Can you work these out from the model? Positions are in its coordinate system, mm. A direction names the side the tool comes from. Give positions to 0.01 mm unless a question says otherwise; leave off trailing zeros. Loops run counter-clockwise (first coordinate to the right, second up) from the corner with the lowest first, then second, coordinate; pieces in that order, holes last.
from build123d import *

# Parameters (mm, degrees)
F0_W     = 173
F0_H     = 30
F1_DEPTH = 3
F2_R     = 9
F3_DEPTH = 15
F4_R     = 2.5
F5_DEPTH = 25
F6_SIZE  = 1
F7_R     = 10
F7_R_2   = 9
F8_DEPTH = 1


with BuildPart() as f1:
    # F0 (on Top) → F1 (new body)
    with BuildSketch(Plane.XY):
        Rectangle(F0_W, F0_H)
    extrude(amount=-F1_DEPTH)

    # F2 (on face) → F3 (join)
    with BuildSketch(Plane.XY):
        with Locations((-67.5, 0.1318904841)):
            Circle(F2_R)
        with Locations((-22.5, 0.1318904841)):
            Circle(F2_R)
        with Locations((22.5, 0.1318904841)):
            Circle(F2_R)
        with Locations((67.5, 0.1318904841)):
            Circle(F2_R)
    extrude(amount=F3_DEPTH)

    # F4 (on face) → F5 (cut)
    with BuildSketch(Plane.XY):
        with Locations((-48.203933984, 0)):
            Circle(F4_R)
        with Locations((48.203933984, 0)):
            Circle(F4_R)
    extrude(amount=-F5_DEPTH, mode=Mode.SUBTRACT)

    # F6
    f6_edges = [f1.edges().sort_by_distance(p)[0] for p in [
        (-50.703934, 0, 0),
        (45.703934, 0, 0),
    ]]
    chamfer(f6_edges, length=F6_SIZE)

    # F7 (on face) → F8 (join, symmetric)
    with BuildSketch(Plane.XY.offset(15)):
        with Locations((-67.5, 0.1318904841)):
            Circle(F7_R)
        with Locations((-67.5, 0.1318904841)):
            Circle(F7_R_2, mode=Mode.SUBTRACT)
        with Locations((-22.5, 0.1318904841)):
            Circle(F7_R)
        with Locations((22.5, 0.1318904841)):
            Circle(F7_R)
        with Locations((67.5, 0.1318904841)):
            Circle(F7_R)
        with Locations((-67.5, 0.1318904841)):
            Circle(F7_R_2)
    extrude(amount=F8_DEPTH, both=True)


solid = f1.part
(1) Which directions (+Z, -Z, +X, -X, +Y, -Y) give clear straight access to the entire face, cutting with the end or side of a thin tool? Please do faces 4 (the flat face through (86.5, 0, -1)), 5 (the cylindrical face through (76.084, 2.835, 6.902)), 6 (the cylindrical face through (-77.49, 0.57, 15.01)).
Returned:
face 4: +Z, -Z, +X, +Y, -Y
face 5: none
face 6: +Z
(2) Will these pins go through, and if not, where does the flat tip stop? P1, Ø6, axis at y = 8.5, z = 10.5, coming from the +X side; P2, Ø15, axis at x = -0.5, y = 5.5, coming from the +Z side; P3, Ø4, axis at x = 25, z = 9, coming from the -Y side.
Returned:
P1: stops at x = 74.72
P2: stops at z = 0
P3: stops at y = -8.85
(3) Suppose I cut it at D-D on x = -29. List the corners of the cut face in (y, z) for me, plus the area to 3 significant figures.
Returned:
outline: (-15, -3) - (15, -3) - (15, 0) - (6.36, 0) - (6.36, 14) - (7.73, 14) - (7.73, 16) - (-7.47, 16) - (-7.47, 14) - (-6.09, 14) - (-6.09, 0) - (-15, 0) - close
area: 295 mm2
(4) Suppose I cut it at B-B on z = 3.5. List the corners of the cut face in (x, y) for me.
Returned:
outline: circle Ø18 at (-67.5, 0.13); circle Ø18 at (-22.5, 0.13); circle Ø18 at (22.5, 0.13); circle Ø18 at (67.5, 0.13)
(5) Suppose I cut it at A-A on x = 22.5. List the corners of the cut face in (y, z) for me.
Returned:
outline: (-15, -3) - (15, -3) - (15, 0) - (9.13, 0) - (9.13, 14) - (10.13, 14) - (10.13, 16) - (-9.87, 16) - (-9.87, 14) - (-8.87, 14) - (-8.87, 0) - (-15, 0) - close
(6) Suppose I cut it at C-C on y = -13. List the corners of the cut face in (x, z) for me.
Returned:
outline: (-86.5, -3) - (86.5, -3) - (86.5, 0) - (-86.5, 0) - close
(7) Thinking about a two-plate mould opening in Z: for faces 1 (the flat face through (-23, 0, 16)), 2 (the cylindrical face through (30.81, -3.32, 6.9)), 3 (the cylindrical face through (-50.7, 0.1, -2)), which applies, pulls with the +Z half, pulls with the -Z half, needs draft (parallel to the pull), parting line crosses it, or undercut?
Returned:
face 1: pulls with the +Z half
face 2: undercut
face 3: needs draft
(8) Please list where these lines run through material, in increasing order: probe 1 along Z at (x, y) = (-51.5, -4.75); probe 2 along X at (y, z) = (5.25, 2); probe 3 along X at (y, z) = (8, 7.5).
Returned:
probe 1: z = -3 to 0
probe 2: x = -74.9 to -60.1, -29.9 to -15.1, 15.1 to 29.9, 60.1 to 74.9
probe 3: x = -71.87 to -63.13, -26.87 to -18.13, 18.13 to 26.87, 63.13 to 71.87
